Part model, mm, in its own coordinate system. Face numbers are marked on the shaded views. A direction names the side the tool comes from. Round coordinates to 2 decimals unless told otherwise and drop trailing zeros. Write each loop counter-clockwise with the first axis right and the second up, starting at its lowest first coordinate (ties: lowest second). Pieces come first, ordered by that corner, then holes.
1) Pull direction Y, two halves, no side cores. Call the marked faces 1, 2, 3 and 4: +Y half, -Y half, draft (parallel to the pull), parting line (faces both ways), or undercut.
2) Saw through at D-D on z = -7.25. Write the cut outline in (x, y).
3) Which spindle directions (+Z, -Z, +X, -X, +Y, -Y) get a long thin tool onto all of the face, cutting with end or side? Do the marked faces 5, 6 and 7. Say none if no direction does.
4) Saw through at A-A on y = -6.5. Write the cut outline in (x, z).
5) Saw through at B-B on x = 6.75. Write the cut outline in (y, z), and give its area (3 significant figures).
6) Saw through at C-C on x = 0. Write the cut outline in (y, z).
7) Drill centre lines: L1, parallel to Y at x = 3, z = 0.75; L2, parallel to Z at x = 0, y = -27.6; L3, parallel to Z at x = 7.5, y = -8.5. Where is each one in solid material? Low to high.
8) Flat gauge pins, fed straight in: pin 1 (2 mm diameter, centred on y = 13.79, z = 0, fed in from -X); pin 2 (1.5 mm diameter, centred on x = 0, y = 26.5, fed in from -Z); pin 3 (3 mm diameter, centred on x = 2, y = 23.5, fed in from -Z). Where does each tip first touch, or does it go through?
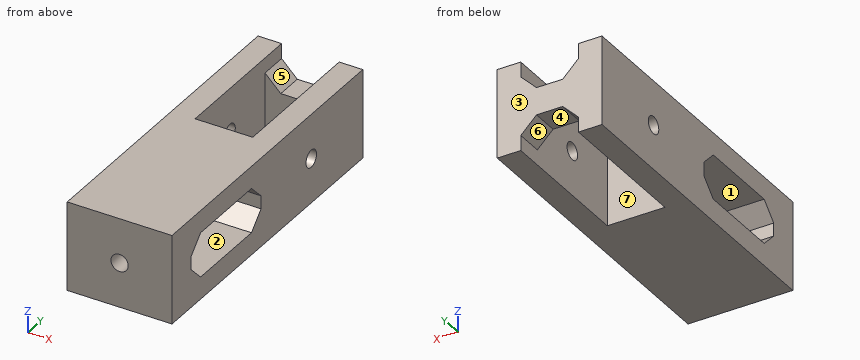
```python
from build123d import *

# Parameters (mm, degrees)
F0_W          = 60
F0_H          = 17
F1_DEPTH      = 10
F2_W          = 22
F2_H          = 8.5
F3_DEPTH      = 25
F4_W          = 11
F4_H          = 22
F5_DEPTH      = 25
F6_R          = 1.65
F7_DEPTH      = 25
F8_W          = 11
F8_H          = 5.8824277986
F9_DEPTH      = 6
F10_SIZE      = 3
F12_DEPTH     = 1.5
F13_R         = 1.65
F14_DEPTH     = 10
F15_T1_DEPTH  = 20
F15_T6_DEPTH  = 20
F15_T12_DEPTH = 20
F15_T18_DEPTH = 20
F15_T25_DEPTH = 20
F15_T31_DEPTH = 20
F15_T37_DEPTH = 20
F15_T43_DEPTH = 20
F15_T49_DEPTH = 20
F15_T56_DEPTH = 20
F15_T62_DEPTH = 20


# Not quite as in the source:
# - a fillet or chamfer that OpenCascade refuses, or shapes differently, is made with other operations: its cross-section is extruded or revolved along the edge and cut away or added


with BuildPart() as f1:
    # F0 (on Right) → F1 (new body, symmetric)
    with BuildSketch(Plane.YZ):
        Rectangle(F0_W, F0_H)
    extrude(amount=F1_DEPTH, both=True)

    # F2 (on face) → F3 (cut)
    with BuildSketch(Plane.YZ.offset(10)):
        with Locations((-13, 0)):
            Rectangle(F2_W, F2_H)
    extrude(amount=-F3_DEPTH, mode=Mode.SUBTRACT)

    # F4 (on face) → F5 (cut)
    with BuildSketch(Plane.XY.offset(8.5)):
        with Locations((0, 13.7926964089)):
            Rectangle(F4_W, F4_H)
    extrude(amount=-F5_DEPTH, mode=Mode.SUBTRACT)

    # F6 (on face) → F7 (cut)
    with BuildSketch(Plane(origin=(-10, 0, 0), x_dir=(0, -1, 0), z_dir=(-1, 0, 0))):
        with Locations((-13.7926964089, 0)):
            Circle(F6_R)
    extrude(amount=-F7_DEPTH, mode=Mode.SUBTRACT)

    # F8 (on face) → F9 (cut)
    with BuildSketch(Plane(origin=(0, 30, 0), x_dir=(-1, 0, 0), z_dir=(0, 1, 0))):
        with Locations((0, 5.5587861007)):
            Rectangle(F8_W, F8_H)
        with Locations((0, -5.5587861007)):
            Rectangle(F8_W, F8_H)
    extrude(amount=-F9_DEPTH, mode=Mode.SUBTRACT)

    # F10
    f10_edges = [f1.edges().sort_by_distance(p)[0] for p in [
        (-5.5, 27.396348, 2.617572),
        (5.5, 27.396348, 2.617572),
        (5.5, 27.396348, -2.617572),
        (-5.5, 27.396348, -2.617572),
    ]]
    chamfer(f10_edges, length=F10_SIZE)

    # F11 (on face) → F12 (cut, symmetric)
    with BuildSketch(Plane(origin=(0, -24, 0), x_dir=(-1, 0, 0), z_dir=(0, 1, 0))):
        Polygon((-1.7320508076, 3), (-3.4641016151, 0), (-1.7320508076, -3), (1.7320508076, -3), (3.4641016151, 0), (1.7320508076, 3), align=None)
    extrude(amount=F12_DEPTH, both=True, mode=Mode.SUBTRACT)

    # F13 (on face) → F14 (cut)
    with BuildSketch(Plane.XZ.offset(30)):
        Circle(F13_R)
    extrude(amount=-F14_DEPTH, mode=Mode.SUBTRACT)

    # F15: chamfer of 3 on 4 edges, made by hand

    # F15_s2 → F15_t1 (join)
    with BuildSketch(Plane.YZ.offset(-10)):
        Polygon((-2, 1.25), (-5, 4.25), (-2, 4.25), align=None)
        Polygon((-5, -4.25), (-2, -1.25), (-2, -4.25), align=None)
    extrude(amount=F15_T1_DEPTH)


with BuildPart() as f15_tool4:
    # F15_s5 → F15_t6 (new body)
    with BuildSketch(Plane.YZ.offset(10)):
        Polygon((-21, -4.25), (-24, -1.25), (-24, -4.25), align=None)
    extrude(amount=-F15_T6_DEPTH)

    split(bisect_by=Plane.XY.offset(-3), keep=Keep.BOTTOM)

    split(bisect_by=Plane(origin=(2.5980762114, 0, -1.5), x_dir=(0, 1, 0), z_dir=(0.8660254038, 0, -0.5)), keep=Keep.TOP)


with BuildPart() as f1_1:
    add(f1.part)

    # F15_t3: union F15_tool4
    add(f15_tool4.part)


with BuildPart() as f15_tool10:
    # F15_s11 → F15_t12 (new body)
    with BuildSketch(Plane.YZ.offset(10)):
        Polygon((-21, -4.25), (-24, -1.25), (-24, -4.25), align=None)
    extrude(amount=-F15_T12_DEPTH)

    split(bisect_by=Plane.XY.offset(-3), keep=Keep.TOP)

    split(bisect_by=Plane(origin=(2.5980762114, 0, -1.5), x_dir=(0, 1, 0), z_dir=(0.8660254038, 0, -0.5)), keep=Keep.TOP)


with BuildPart() as f1_2:
    add(f1_1.part)

    # F15_t9: union F15_tool10
    add(f15_tool10.part)


with BuildPart() as f15_tool16:
    # F15_s17 → F15_t18 (new body)
    with BuildSketch(Plane.YZ.offset(10)):
        Polygon((-21, -4.25), (-24, -1.25), (-24, -4.25), align=None)
    extrude(amount=-F15_T18_DEPTH)

    split(bisect_by=Plane(origin=(-2.5980762114, 0, -1.5), x_dir=(0, 1, 0), z_dir=(0.8660254038, 0, 0.5)), keep=Keep.TOP)

    split(bisect_by=Plane.XY.offset(-3), keep=Keep.BOTTOM)

    split(bisect_by=Plane(origin=(2.5980762114, 0, -1.5), x_dir=(0, 1, 0), z_dir=(-0.8660254038, 0, 0.5)), keep=Keep.TOP)


with BuildPart() as f1_3:
    add(f1_2.part)

    # F15_t15: union F15_tool16
    add(f15_tool16.part)


with BuildPart() as f15_tool23:
    # F15_s24 → F15_t25 (new body)
    with BuildSketch(Plane.YZ.offset(10)):
        Polygon((-21, -4.25), (-24, -1.25), (-24, -4.25), align=None)
    extrude(amount=-F15_T25_DEPTH)

    split(bisect_by=Plane(origin=(-2.5980762114, 0, -1.5), x_dir=(0, 1, 0), z_dir=(-0.8660254038, 0, -0.5)), keep=Keep.TOP)

    split(bisect_by=Plane.XY.offset(-3), keep=Keep.BOTTOM)


with BuildPart() as f1_4:
    add(f1_3.part)

    # F15_t22: union F15_tool23
    add(f15_tool23.part)


with BuildPart() as f15_tool29:
    # F15_s30 → F15_t31 (new body)
    with BuildSketch(Plane.YZ.offset(10)):
        Polygon((-21, -4.25), (-24, -1.25), (-24, -4.25), align=None)
    extrude(amount=-F15_T31_DEPTH)

    split(bisect_by=Plane(origin=(-2.5980762114, 0, -1.5), x_dir=(0, 1, 0), z_dir=(-0.8660254038, 0, -0.5)), keep=Keep.TOP)

    split(bisect_by=Plane.XY.offset(-3), keep=Keep.TOP)


with BuildPart() as f1_5:
    add(f1_4.part)

    # F15_t28: union F15_tool29
    add(f15_tool29.part)


with BuildPart() as f15_tool35:
    # F15_s36 → F15_t37 (new body)
    with BuildSketch(Plane.YZ.offset(10)):
        Polygon((-24, 1.25), (-21, 4.25), (-24, 4.25), align=None)
    extrude(amount=-F15_T37_DEPTH)

    split(bisect_by=Plane(origin=(2.5980762114, 0, 1.5), x_dir=(0, 1, 0), z_dir=(0.8660254038, 0, 0.5)), keep=Keep.TOP)

    split(bisect_by=Plane.XY.offset(3), keep=Keep.BOTTOM)


with BuildPart() as f1_6:
    add(f1_5.part)

    # F15_t34: union F15_tool35
    add(f15_tool35.part)


with BuildPart() as f15_tool41:
    # F15_s42 → F15_t43 (new body)
    with BuildSketch(Plane.YZ.offset(10)):
        Polygon((-24, 1.25), (-21, 4.25), (-24, 4.25), align=None)
    extrude(amount=-F15_T43_DEPTH)

    split(bisect_by=Plane(origin=(2.5980762114, 0, 1.5), x_dir=(0, 1, 0), z_dir=(0.8660254038, 0, 0.5)), keep=Keep.TOP)

    split(bisect_by=Plane.XY.offset(3), keep=Keep.TOP)


with BuildPart() as f1_7:
    add(f1_6.part)

    # F15_t40: union F15_tool41
    add(f15_tool41.part)


with BuildPart() as f15_tool47:
    # F15_s48 → F15_t49 (new body)
    with BuildSketch(Plane.YZ.offset(10)):
        Polygon((-24, 1.25), (-21, 4.25), (-24, 4.25), align=None)
    extrude(amount=-F15_T49_DEPTH)

    split(bisect_by=Plane(origin=(-2.5980762114, 0, 1.5), x_dir=(0, 1, 0), z_dir=(0.8660254038, 0, -0.5)), keep=Keep.TOP)

    split(bisect_by=Plane(origin=(2.5980762114, 0, 1.5), x_dir=(0, 1, 0), z_dir=(-0.8660254038, 0, -0.5)), keep=Keep.TOP)

    split(bisect_by=Plane.XY.offset(3), keep=Keep.TOP)


with BuildPart() as f1_8:
    add(f1_7.part)

    # F15_t46: union F15_tool47
    add(f15_tool47.part)


with BuildPart() as f15_tool54:
    # F15_s55 → F15_t56 (new body)
    with BuildSketch(Plane.YZ.offset(10)):
        Polygon((-24, 1.25), (-21, 4.25), (-24, 4.25), align=None)
    extrude(amount=-F15_T56_DEPTH)

    split(bisect_by=Plane(origin=(-2.5980762114, 0, 1.5), x_dir=(0, 1, 0), z_dir=(-0.8660254038, 0, 0.5)), keep=Keep.TOP)

    split(bisect_by=Plane.XY.offset(3), keep=Keep.BOTTOM)


with BuildPart() as f1_9:
    add(f1_8.part)

    # F15_t53: union F15_tool54
    add(f15_tool54.part)


with BuildPart() as f15_tool60:
    # F15_s61 → F15_t62 (new body)
    with BuildSketch(Plane.YZ.offset(10)):
        Polygon((-24, 1.25), (-21, 4.25), (-24, 4.25), align=None)
    extrude(amount=-F15_T62_DEPTH)

    split(bisect_by=Plane(origin=(-2.5980762114, 0, 1.5), x_dir=(0, 1, 0), z_dir=(-0.8660254038, 0, 0.5)), keep=Keep.TOP)

    split(bisect_by=Plane.XY.offset(3), keep=Keep.TOP)


with BuildPart() as f1_10:
    add(f1_9.part)

    # F15_t59: union F15_tool60
    add(f15_tool60.part)


solid = f1_10.part
```
Completed:
1. face 1: undercut
1. face 2: undercut
1. face 3: +Y half
1. face 4: draft
2. outline: (-10, -30) - (10, -30) - (10, 30) - (5.5, 30) - (5.5, 2.79) - (-5.5, 2.79) - (-5.5, 30) - (-10, 30) - close
3. face 5: +Z, +Y
3. face 6: -Z, +Y
3. face 7: +Z, -Z
4. outline: (-10, -8.5) - (10, -8.5) - (10, -4.25) - (-10, -4.25) - close; (-10, 4.25) - (10, 4.25) - (10, 8.5) - (-10, 8.5) - close
5. outline: (-30, -8.5) - (30, -8.5) - (30, 8.5) - (-30, 8.5) - close; hole (-24, -1.25) - (-21, -4.25) - (-5, -4.25) - (-2, -1.25) - (-2, 1.25) - (-5, 4.25) - (-21, 4.25) - (-24, 1.25) - close; hole circle Ø3.3 at (13.79, 0)
5. area: 842 mm2
6. outline: (-30, -8.5) - (2.79, -8.5) - (2.79, 8.5) - (-30, 8.5) - (-30, 1.65) - (-25.5, 1.65) - (-25.5, 3) - (-22.25, 3) - (-21, 4.25) - (-5, 4.25) - (-2, 1.25) - (-2, -1.25) - (-5, -4.25) - (-21, -4.25) - (-22.25, -3) - (-25.5, -3) - (-25.5, -1.65) - (-30, -1.65) - close; (24.79, -2.62) - (30, -2.62) - (30, 2.62) - (24.79, 2.62) - close
7. L1: y = -30 to -25.5, -2 to 2.79, 24.79 to 30
7. L2: z = -8.5 to -1.65, 1.65 to 8.5
7. L3: z = -8.5 to -4.25, 4.25 to 8.5
8. pin 1: passes through
8. pin 2: stops at z = -2.62
8. pin 3: stops at z = -2.88
